Check sheet for the drawn part. Datum: minimum x, y, z corner. Units: mm. Give positions to 0.01 mm unless a question says otherwise; leave off trailing zeros. Loops run counter-clockwise (first coordinate to the right, second up) from the corner with the lowest first, then second, coordinate; pieces in that order, holes last.
1. Cross-section at C-C, the plane y = 9.75. Record the cut outline in (x, z).
2. Release check for a two-part mould opening along Z. For the marked faces 1, 2 and 3 record: +Z half, -Z half, draft (parallel to the pull), parting line (faces both ways), or undercut.
3. Cross-section at A-A, the plane y = 4.5. Record the cut outline in (x, z).
4. Cross-section at B-B, the plane y = 16.25. Record the cut outline in (x, z).
5. Material ranges on L1, parallel to Z at x = 30, y = 2.5; L2, parallel to Z at x = 26, y = 5.5 (1 decimal); L3, parallel to Y at x = 51.5, z = 15.5, recorded low to high.
6. Go/stop test with flat-tipped pins: pin 1 Ø10 at (x, y) = (53.5, 2.5) entering from -Z; pin 2 Ø4.5 at (y, z) = (15, 30.5) entering from +X; pin 3 Ø6.5 at (x, z) = (30, 30) entering from -Y. Record where each tip stops, or that it passes through.
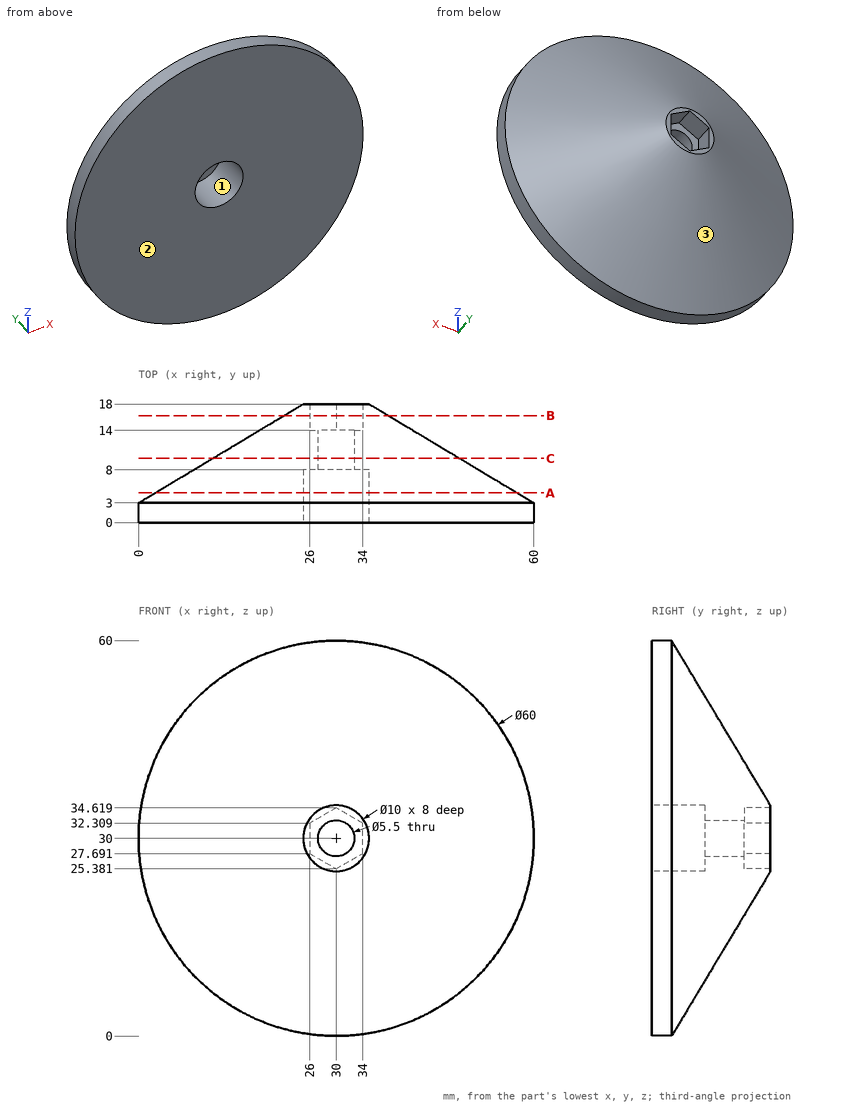
Result:
1. outline: circle Ø37.5 at (30, 30); hole circle Ø5.5 at (30, 30)
2. face 1: undercut
2. face 2: draft
2. face 3: parting line
3. outline: circle Ø55 at (30, 30); hole circle Ø10 at (30, 30)
4. outline: circle Ø15.83 at (30, 30); hole (26, 27.69) - (30, 25.38) - (34, 27.69) - (34, 32.31) - (30, 34.62) - (26, 32.31) - close
5. L1: z = 0 to 25, 35 to 60
5. L2: z = 4.5 to 27, 33 to 55.5
5. L3: y = 0 to 5.44
6. pin 1: stops at z = 6.38
6. pin 2: stops at x = 43.74
6. pin 3: stops at y = 8
